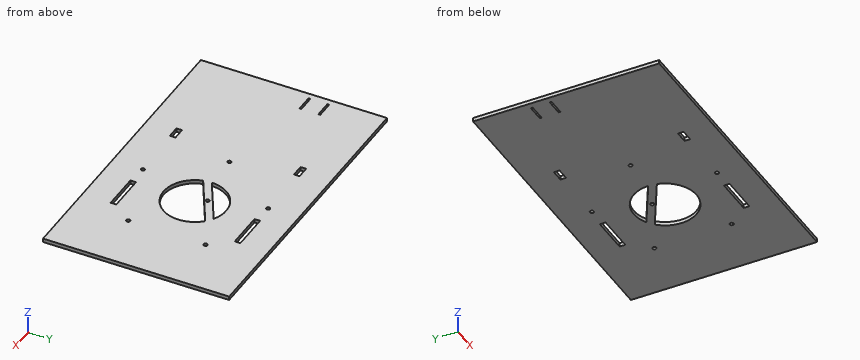
```python
from build123d import *

# Parameters (mm, degrees)
SKETCH1_W           = 240.000854432
SKETCH1_H           = 148.499462854
SKETCH1_R           = 25
SKETCH1_W_2         = 13.501501462
SKETCH1_H_2         = 1.500166829
SKETCH1_H_3         = 1.501200358
SKETCH1_W_3         = 9.930659991
SKETCH1_H_4         = 4.500500488
SKETCH1_W_4         = 29.999719231
SKETCH1_H_5         = 4.500500487
SKETCH1_W_5         = 30.000235995
BOSS_EXTRUDE2_DEPTH = 3
SKETCH2_R           = 1.5
BOSS_EXTRUDE3_DEPTH = 3
SKETCH3_R           = 1.5
CUT_EXTRUDE1_DEPTH  = 3
SKETCH3_3_R         = 1.5
CUT_EXTRUDE2_DEPTH  = 3


with BuildPart() as part:
    # Sketch1 → Boss-Extrude2 (new body)
    with BuildSketch(Plane.XY):
        Rectangle(SKETCH1_W, SKETCH1_H)
        with Locations((30.570227043, 0.001291911)):
            Circle(SKETCH1_R, mode=Mode.SUBTRACT)
        with Locations((-108.180218479, 30.002561435)):
            Rectangle(SKETCH1_W_2, SKETCH1_H_2, mode=Mode.SUBTRACT)
        with Locations((-108.180218479, 15.00037638)):
            Rectangle(SKETCH1_W_2, SKETCH1_H_3, mode=Mode.SUBTRACT)
        with Locations((-34.96659952, 49.499562569)):
            Rectangle(SKETCH1_W_3, SKETCH1_H_4, mode=Mode.SUBTRACT)
        with Locations((44.998545318, 49.499562569)):
            Rectangle(SKETCH1_W_4, SKETCH1_H_4, mode=Mode.SUBTRACT)
        with Locations((-34.96659952, -49.498529041)):
            Rectangle(SKETCH1_W_3, SKETCH1_H_5, mode=Mode.SUBTRACT)
        with Locations((45.000353993, -49.498529041)):
            Rectangle(SKETCH1_W_5, SKETCH1_H_5, mode=Mode.SUBTRACT)
    extrude(amount=BOSS_EXTRUDE2_DEPTH)

    # Sketch2 → Boss-Extrude3 (add)
    # profile 1 of 2: a face of its own
    with BuildSketch(Plane.XY.offset(3)):
        with Locations((45.531251612, -26.95033278)):
            Circle(SKETCH2_R)
    # profile 2 of 2: a face of its own
    with BuildSketch(Plane.XY.offset(3)):
        Polygon((27.163645512, 5.615664927), (48.357135802, 17.569042957), (45.390356123, 22.829180815), (3.83834926, -0.606640239), (6.127103067, -6.249192671), align=None)
        with Locations((25.948903296, 7.769418226)):
            Circle(SKETCH2_R, mode=Mode.SUBTRACT)
    extrude(amount=-BOSS_EXTRUDE3_DEPTH)

    # Sketch3 → Cut-Extrude1 (cut)
    with BuildSketch(Plane.XY.offset(3)):
        with Locations((-21.929772957, 0.001291911)):
            Circle(SKETCH3_R)
    extrude(amount=-CUT_EXTRUDE1_DEPTH, mode=Mode.SUBTRACT)

    # Sketch3<3> → Cut-Extrude2 (cut)
    with BuildSketch(Plane.XY.offset(3)):
        with Locations((-21.929772957, 0.001291911)):
            Circle(SKETCH3_3_R)
        with Locations((14.346834838, 49.931759016)):
            Circle(SKETCH3_3_R)
        with Locations((73.043619248, 30.860017656)):
            Circle(SKETCH3_3_R)
        with Locations((73.043619248, -30.857433835)):
            Circle(SKETCH3_3_R)
        with Locations((14.346834838, -49.929175195)):
            Circle(SKETCH3_3_R)
    extrude(amount=-CUT_EXTRUDE2_DEPTH, mode=Mode.SUBTRACT)


solid = part.part
```
Geometry check sheet. Reference: the model listing, model coordinates, mm. Round coordinates to 2 decimals unless told otherwise and drop trailing zeros. Loops run counter-clockwise (first coordinate to the right, second up) from the corner with the lowest first, then second, coordinate; pieces in that order, holes last. Notation, with made-up numbers: M 22,47.5 L 69,47.5 A16 ccw 69,61.5 Z; hole C 29.5,-38.75 d7. An arc over 180 degrees is marked long. Return JSON: item names as keys, results as strings. Group by question number.
(1) Section check A-A, the plane x = 39.5. Enter the section's corners in (y, z), and give its area (3 significant figures).
(2) Scan lines: line 1 along X through (y, z) = (50, 0.95); line 2 along Y through (x, z) = (-102.5, 1.2); line 3 along Y through (x, z) = (59, 1.55). Record each from-to range of solid material in increasing order. Write a range as [from, to].
(3) Section check B-B, the plane x = 10. Enter the section's corners in (y, z).
(4) Section check C-C, the plane z = 0.7. Give the number of separate pieces and of enclosed holes in the cut face, and give its area (3 significant figures).
(5) Go/stop test with flat-tipped pins: pin 1 (2 mm diameter, centred on x = 36.5, y = 29.5, fed in from -Z); pin 2 (1.8 mm diameter, centred on x = 73.04, y = -30.86, fed in from +Z). Record where each tip stops, or that it passes through.
Data:
{
 "1": {"outline": "M -74.25,0 L -51.75,0 L -51.75,3 L -74.25,3 Z; M -47.25,0 L -23.35,0 L -23.35,3 L -47.25,3 Z; M 12.57,0 L 19.51,0 L 19.51,3 L 12.57,3 Z; M 23.35,0 L 47.25,0 L 47.25,3 L 23.35,3 Z; M 51.75,0 L 74.25,0 L 74.25,3 L 51.75,3 Z", "area": "299 mm²"},
 "2": {"line 1": "[-120, -39.93], [-30, 12.85], [15.85, 30], [60, 120]", "line 2": "[-74.25, 14.25], [15.75, 29.25], [30.75, 74.25]", "line 3": "[-74.25, -51.75], [-47.25, 47.25], [51.75, 74.25]"},
 "3": {"outline": "M -74.25,0 L -14.21,0 L -14.21,3 L -74.25,3 Z; M -4.06,0 L 2.87,0 L 2.87,3 L -4.06,3 Z; M 14.21,0 L 74.25,0 L 74.25,3 L 14.21,3 Z"},
 "4": {"separate pieces": "1", "enclosed holes": "14", "area": "33,500 mm²"},
 "5": {"pin 1": "z = 0", "pin 2": "through"}
}
